Build history of the part. All positions in model axes, mm. Face numbers are marked on the shaded views. A direction names the side the tool comes from. Round coordinates to 2 decimals unless told otherwise and drop trailing zeros. Write each loop counter-clockwise with the first axis right and the second up, starting at its lowest first coordinate (ties: lowest second). Pieces come first, ordered by that corner, then holes.
1) Wall check: probe 1 along X at (y, z) = (4.85, 0); probe 2 along X at (y, z) = (0.6, -7.5); probe 3 along Z at (x, y) = (51, 5.5). Give the ranges that are in metal, low to high.
2) Which spindle directions (+Z, -Z, +X, -X, +Y, -Y) get a long thin tool onto all of the face, cutting with end or side? Do the marked faces 1, 2 and 3. Say none if no direction does.
3) Saw through at A-A (y = 5.25). Write the cut outline in (x, z), plus the area to 3 significant figures.
4) Saw through at B-B (z = -51). Write the cut outline in (x, y), plus the area to 3 significant figures.
5) Saw through at D-D (z = 0). State how many separate pieces and enclosed holes the cut face has, plus the area to 3 significant figures.
6) Flat gauge pins, fed straight in: pin 1 (1.5 mm diameter, centred on x = 0, z = 4.5, fed in from +Y); pin 2 (18.5 mm diameter, centred on x = -25, z = -2, fed in from +Y); pin 3 (5.5 mm diameter, centred on x = 0, z = 7.5, fed in from +Y). Where does each tip first touch, or does it go through?
7) Pull direction Z, two halves, no side cores. Call the marked faces 4, 5 and 6: +Z half, -Z half, draft (parallel to the pull), parting line (faces both ways), or undercut.
from build123d import *
from OCP.BRepFilletAPI import BRepFilletAPI_MakeFillet

# Parameters (mm, degrees)
MOUNTING_BASE_DEPTH                             = 4.064
LOAD_CELL_ARMS_DEPTH                            = 4.064
M4_CLEARANCE_HOLE1_D                            = 4.3
FILLET1_R1                                      = 3.175
FILLET1_R2                                      = 1.5875
SKETCH15_R                                      = 4.65
SKETCH15_R_2                                    = 2.15
BOSS_EXTRUDE2_DEPTH                             = 3
SKETCH12_OUTSIDE_W                              = 165.308
SKETCH12_OUTSIDE_H                              = 165.308
SKETCH12_OUTSIDE_W_2                            = 115
SKETCH12_OUTSIDE_H_2                            = 115
CUT_EXTRUDE2_DEPTH                              = 20
CSK_FOR_M3_FLAT_HEAD_MACHINE_SCREW1_D           = 3.4
CSK_FOR_M3_FLAT_HEAD_MACHINE_SCREW1_CSINK_D     = 6.3
CSK_FOR_M3_FLAT_HEAD_MACHINE_SCREW1_CSINK_ANGLE = 90
SKETCH14_W                                      = 20
SKETCH14_H                                      = 20
CUT_EXTRUDE3_DEPTH                              = 1.5
CUT_EXTRUDE4_START                              = -4.064
SKETCH14_2_W                                    = 20
SKETCH14_2_H                                    = 20
CUT_EXTRUDE4_DEPTH                              = 1.5
FILLET2_R                                       = 1.5


with BuildPart() as part:
    # Sketch1 → Mounting base (new body)
    with BuildSketch(Plane(origin=(0, 0, 0), x_dir=(1, 0, 0), z_dir=(0, 1, 0))):
        Polygon((-63.639610307, 0), (0, -63.639610307), (63.639610307, 0), (0, 63.639610307), align=None)
        Polygon((-49.497474683, 0), (0, 49.497474683), (49.497474683, 0), (0, -49.497474683), align=None, mode=Mode.SUBTRACT)
    extrude(amount=MOUNTING_BASE_DEPTH)

    # Sketch2 → load cell arms (add, through all)
    with BuildSketch(Plane(origin=(0, 4.064, 0), x_dir=(1, 0, 0), z_dir=(0, 1, 0))):
        Polygon((-49.497474683, 10), (-49.497474683, -10), (-10, -10), (-10, -49.497474683), (10, -49.497474683), (10, -10), (49.497474683, -10), (49.497474683, 10), (10, 10), (10, 49.497474683), (-10, 49.497474683), (-10, 10), align=None)
    extrude(amount=-LOAD_CELL_ARMS_DEPTH)

    # M4 Clearance Hole1 (through all)
    with Locations(Plane(origin=(0, 4.064, 0), x_dir=(1, 0, 0), z_dir=(0, 1, 0))):
        with Locations((-51, 0), (0, 51), (51, 0), (0, -51)):
            Hole(M4_CLEARANCE_HOLE1_D / 2)

    # Fillet1: one fillet with a radius per group of edges: ONE call of the kernel's fillet builder (fillet() takes one radius for all edges)
    fillet1_edges_1 = [part.edges().sort_by_distance(p)[0] for p in [
        (-10, 2.032, 10),
        (-10, 2.032, -10),
        (10, 2.032, -10),
        (10, 2.032, 10),
    ]]
    fillet1_edges_2 = [part.edges().sort_by_distance(p)[0] for p in [
        (-39.497474683, 2.032, -10),
        (-39.497474683, 2.032, 10),
        (-10, 2.032, 39.497474683),
        (10, 2.032, 39.497474683),
        (39.497474683, 2.032, 10),
        (39.497474683, 2.032, -10),
        (10, 2.032, -39.497474683),
        (-10, 2.032, -39.497474683),
    ]]
    fillet1 = BRepFilletAPI_MakeFillet(part.part.solid().wrapped)
    for e in fillet1_edges_1:
        fillet1.Add(FILLET1_R1, e.wrapped)
    for e in fillet1_edges_2:
        fillet1.Add(FILLET1_R2, e.wrapped)
    add(Compound.cast(fillet1.Shape()), mode=Mode.REPLACE)

    # Sketch15 → Boss-Extrude2 (add)
    # profile 1 of 4: a face of its own
    with BuildSketch(Plane(origin=(0, 4.064, 0), x_dir=(1, 0, 0), z_dir=(0, 1, 0))):
        with Locations(Location((0, -51, 0), (0, 0, 90))):
            Circle(SKETCH15_R)
        with Locations(Location((0, -51, 0), (0, 0, 270))):
            Circle(SKETCH15_R_2, mode=Mode.SUBTRACT)
    # profile 2 of 4: a face of its own
    with BuildSketch(Plane(origin=(0, 4.064, 0), x_dir=(1, 0, 0), z_dir=(0, 1, 0))):
        with Locations(Location((-51, 0, 0), (0, 0, 90))):
            Circle(SKETCH15_R)
        with Locations(Location((-51, 0, 0), (0, 0, 270))):
            Circle(SKETCH15_R_2, mode=Mode.SUBTRACT)
    # profile 3 of 4: a face of its own
    with BuildSketch(Plane(origin=(0, 4.064, 0), x_dir=(1, 0, 0), z_dir=(0, 1, 0))):
        with Locations(Location((0, 51, 0), (0, 0, 90))):
            Circle(SKETCH15_R)
        with Locations(Location((0, 51, 0), (0, 0, 270))):
            Circle(SKETCH15_R_2, mode=Mode.SUBTRACT)
    # profile 4 of 4: a face of its own
    with BuildSketch(Plane(origin=(0, 4.064, 0), x_dir=(1, 0, 0), z_dir=(0, 1, 0))):
        with Locations(Location((51, 0, 0), (0, 0, 90))):
            Circle(SKETCH15_R)
        with Locations(Location((51, 0, 0), (0, 0, 270))):
            Circle(SKETCH15_R_2, mode=Mode.SUBTRACT)
    extrude(amount=BOSS_EXTRUDE2_DEPTH)

    # Sketch12 outside → Cut-Extrude2 (cut)
    with BuildSketch(Plane(origin=(0, 0, 0), x_dir=(1, 0, 0), z_dir=(0, 1, 0))):
        Rectangle(SKETCH12_OUTSIDE_W, SKETCH12_OUTSIDE_H)
        Rectangle(SKETCH12_OUTSIDE_W_2, SKETCH12_OUTSIDE_H_2, mode=Mode.SUBTRACT)
    extrude(amount=CUT_EXTRUDE2_DEPTH, mode=Mode.SUBTRACT)

    # CSK for M3 Flat Head Machine Screw1 (through all)
    with Locations(Plane(origin=(0, 4.064, -7.5), x_dir=(0, 0, 1), z_dir=(0, 1, 0))):
        with Locations((0, 0), (7.5, 7.5), (15, 0), (7.5, -7.5)):
            CounterSinkHole(CSK_FOR_M3_FLAT_HEAD_MACHINE_SCREW1_D / 2, CSK_FOR_M3_FLAT_HEAD_MACHINE_SCREW1_CSINK_D / 2, counter_sink_angle=CSK_FOR_M3_FLAT_HEAD_MACHINE_SCREW1_CSINK_ANGLE)

    # Sketch14 → Cut-Extrude3 (cut)
    with BuildSketch(Plane(origin=(0, 4.064, 0), x_dir=(1, 0, 0), z_dir=(0, 1, 0))):
        with Locations((-25, 0)):
            Rectangle(SKETCH14_W, SKETCH14_H)
        with Locations((0, 25)):
            Rectangle(SKETCH14_W, SKETCH14_H)
        with Locations((25, 0)):
            Rectangle(SKETCH14_W, SKETCH14_H)
        with Locations((0, -25)):
            Rectangle(SKETCH14_W, SKETCH14_H)
    extrude(amount=-CUT_EXTRUDE3_DEPTH, mode=Mode.SUBTRACT)

    # Sketch14<2> → Cut-Extrude4 (cut)
    with BuildSketch(Plane(origin=(0, 4.064, 0), x_dir=(1, 0, 0), z_dir=(0, 1, 0)).offset(CUT_EXTRUDE4_START)):
        with Locations((-25, 0)):
            Rectangle(SKETCH14_2_W, SKETCH14_2_H)
        with Locations((0, 25)):
            Rectangle(SKETCH14_2_W, SKETCH14_2_H)
        with Locations((25, 0)):
            Rectangle(SKETCH14_2_W, SKETCH14_2_H)
        with Locations((0, -25)):
            Rectangle(SKETCH14_2_W, SKETCH14_2_H)
    extrude(amount=CUT_EXTRUDE4_DEPTH, mode=Mode.SUBTRACT)

    # Fillet2
    fillet2_edges = [part.edges().sort_by_distance(p)[0] for p in [
        (0, 2.564, 35),
        (0, 2.564, 15),
        (0, 1.5, 15),
        (0, 1.5, 35),
        (15, 1.5, 0),
        (35, 1.5, 0),
        (0, 1.5, -15),
        (-15, 1.5, 0),
        (-35, 1.5, 0),
        (0, 1.5, -35),
        (15, 2.564, 0),
        (35, 2.564, 0),
        (0, 2.564, -35),
        (0, 2.564, -15),
        (-15, 2.564, 0),
        (-35, 2.564, 0),
    ]]
    fillet(fillet2_edges, radius=FILLET2_R - 0.0001)  # a hair under: the kernel refuses the full size


solid = part.part
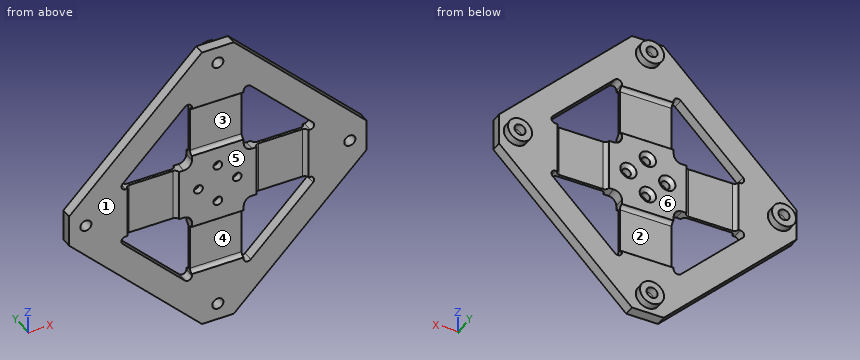
Evaluation:
1. probe 1: x = -55.65 to -53.15, -48.85 to -46.35, 46.35 to 48.85, 53.15 to 55.65
1. probe 2: x = -56.14 to -34.87, -15.13 to -1.7, 1.7 to 15.13, 34.87 to 56.14
1. probe 3: z = -4.65 to -2.15, 2.15 to 4.65
2. face 1: +Z, -Z, +X, -X, -Y
2. face 2: +Y
2. face 3: -Y
3. outline: circle Ø9.3 at (-51, 0); circle Ø9.3 at (0, -51); circle Ø9.3 at (0, 51); circle Ø9.3 at (51, 0); hole circle Ø4.3 at (-51, 0); hole circle Ø4.3 at (0, -51); hole circle Ø4.3 at (0, 51); hole circle Ø4.3 at (51, 0)
3. area: 214 mm2
4. outline: (-12.64, 0) - (-2.15, 0) - (-2.15, 7.06) - (-4.65, 7.06) - (-4.65, 4.06) - (-12.64, 4.06) - close; (2.15, 0) - (12.64, 0) - (12.64, 4.06) - (4.65, 4.06) - (4.65, 7.06) - (2.15, 7.06) - close
4. area: 100 mm2
5. separate pieces: 5
5. enclosed holes: 0
5. area: 314 mm2
6. pin 1: stops at y = 4.06
6. pin 2: stops at y = 2.76
6. pin 3: stops at y = 3.66
7. face 4: undercut
7. face 5: draft
7. face 6: undercut
